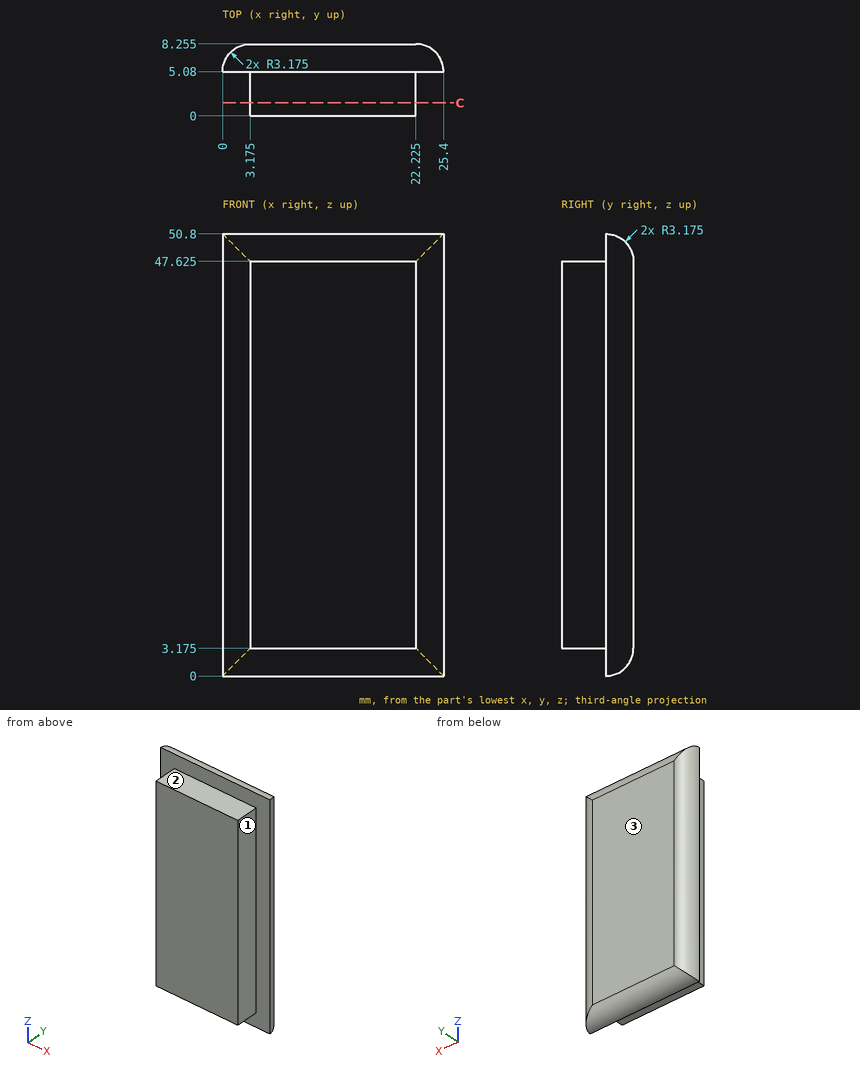
Design review of the part shown in the three views and the two pictorial views. Dimensions are in mm from the part's minimum x, y and z. A direction names the side the tool comes from. Round coordinates to 2 decimals unless told otherwise and drop trailing zeros. Write each loop counter-clockwise with the first axis right and the second up, starting at its lowest first coordinate (ties: lowest second). Pieces come first, ordered by that corner, then holes.
Item 1: Clearance check with flat-ended pins moving along their axes: pin 1 Ø1.5 at (x, y) = (15, 2) entering from +Z (3 decimals); pin 2 Ø1.5 at (y, z) = (1.5, 15) entering from -X (3 decimals); pin 3 Ø1 at (y, z) = (7, 28) entering from -X (3 decimals). State where each tip first meets the part, or that it passes through.
Item 2: We need section C-C on y = 1.5. Write out the cut boundary in (x, z) (3 decimals), and give its area (3 significant figures).
Item 3: For probe 1 along Z at (x, y) = (10.25, 1) (3 decimals); probe 2 along X at (y, z) = (1.75, 13.5) (3 decimals); probe 3 along Y at (x, z) = (3, 26), list the stretches that pass through material, from the lowest coordinate up.
Item 4: For the marked faces 1, 2 and 3, list the 3-axis set-ups (+Z, -Z, +X, -X, +Y, -Y) from which the entire face can be reached by the end or side of a thin tool; tool diameter is ignored.
Returned:
1. pin 1: stops at z = 47.625
1. pin 2: stops at x = 3.175
1. pin 3: stops at x = 0.335
2. outline: (3.175, 3.175) - (22.225, 3.175) - (22.225, 47.625) - (3.175, 47.625) - close
2. area: 847 mm2
3. probe 1: z = 3.175 to 47.625
3. probe 2: x = 3.175 to 22.225
3. probe 3: y = 5.08 to 8.25
4. face 1: +Z, -Z, +X, -Y
4. face 2: +Z, +X, -X, -Y
4. face 3: +Z, -Z, +X, -X, +Y
